The listing builds one solid part. Answer for the finished solid, in the listing's coordinates (mm). A direction names the side the tool comes from. Give positions to 0.01 mm unless a question says otherwise; leave off trailing zeros. Loops run counter-clockwise (first coordinate to the right, second up) from the corner with the lowest first, then second, coordinate; pieces in that order, holes last. Notation, with made-up numbers: (-14.75, 4) -> (22.25, 4) arc R13 ccw to (22.25, 25) -> close; hole circle Ø8 at (23, 9.5). An arc over 180 degrees is marked (long way). One line per question, with ' | ' between items. Start each with the question number.
from build123d import *
from OCP.BRepFilletAPI import BRepFilletAPI_MakeChamfer

# Parameters (mm, degrees)
SKETCH1_W           = 11.3
SKETCH1_H           = 9.85
BOSS_EXTRUDE1_DEPTH = 15.75
SKETCH2_W           = 0.45
SKETCH2_H           = 4
CUT_EXTRUDE1_DEPTH  = 15.75
SKETCH3_W           = 5.6
SKETCH3_H           = 3.18
CUT_EXTRUDE2_DEPTH  = 8.38
CHAMFER1_SIZE       = 0.38
CHAMFER1_SIZE2      = 0.219393102
CHAMFER2_SIZE       = 0.38
CHAMFER2_SIZE2      = 0.219393102
SKETCH4_W           = 1
SKETCH4_H           = 10.13
SKETCH4_H_2         = 8.63
BOSS_EXTRUDE2_DEPTH = 0.83
SKETCH5_W           = 1.2
SKETCH5_H           = 0.75
CUT_EXTRUDE3_DEPTH  = 19.829431749
SKETCH6_W           = 1.2
SKETCH6_H           = 6.44
CUT_EXTRUDE4_DEPTH  = 1.29
CUT_EXTRUDE5_DEPTH  = 2


with BuildPart() as part:
    # Sketch1 → Boss-Extrude1 (new body)
    with BuildSketch(Plane.XY.offset(-0.38)):
        with Locations((0, 5.325)):
            Rectangle(SKETCH1_W, SKETCH1_H)
    extrude(amount=-BOSS_EXTRUDE1_DEPTH)

    # Sketch2 → Cut-Extrude1 (cut)
    with BuildSketch(Plane(origin=(0, 10.25, 0), x_dir=(1, 0, 0), z_dir=(0, 1, 0))):
        with Locations((-5.425, 14.13)):
            Rectangle(SKETCH2_W, SKETCH2_H)
        with Locations((5.425, 14.13)):
            Rectangle(SKETCH2_W, SKETCH2_H)
    extrude(amount=-CUT_EXTRUDE1_DEPTH, mode=Mode.SUBTRACT)

    # Sketch3 → Cut-Extrude2 (cut)
    with BuildSketch(Plane.XY.offset(-0.38)):
        with BuildLine():
            Line((-4.225, 7.352598846), (-4.225, 6.45))
            Line((-4.225, 6.45), (-4.625, 6.45))
            Line((-4.625, 6.45), (-4.625, 2.45))
            Line((-4.625, 2.45), (-4.225, 2.45))
            Line((-4.225, 2.45), (-4.225, 1.74))
            ThreePointArc((-4.225, 1.74), (-4.113700577, 1.471299423), (-3.845, 1.36))
            Line((-3.845, 1.36), (3.845, 1.36))
            ThreePointArc((3.845, 1.36), (4.113700577, 1.471299423), (4.225, 1.74))
            Line((4.225, 1.74), (4.225, 2.45))
            Line((4.225, 2.45), (4.625, 2.45))
            Line((4.625, 2.45), (4.625, 6.45))
            Line((4.625, 6.45), (4.225, 6.45))
            Line((4.225, 6.45), (4.225, 7.352598846))
            ThreePointArc((4.225, 7.352598846), (4.196074222, 7.498018551), (4.113700577, 7.621299423))
            Line((4.113700577, 7.621299423), (2.706299423, 9.028700577))
            ThreePointArc((2.706299423, 9.028700577), (2.583018551, 9.111074222), (2.437598846, 9.14))
            Line((2.437598846, 9.14), (-2.437598846, 9.14))
            ThreePointArc((-2.437598846, 9.14), (-2.583018551, 9.111074222), (-2.706299423, 9.028700577))
            Line((-2.706299423, 9.028700577), (-4.113700577, 7.621299423))
            ThreePointArc((-4.113700577, 7.621299423), (-4.196074222, 7.498018551), (-4.225, 7.352598846))
        make_face()
        with Locations((0, 5.25)):
            Rectangle(SKETCH3_W, SKETCH3_H, mode=Mode.SUBTRACT)
    extrude(amount=-CUT_EXTRUDE2_DEPTH, mode=Mode.SUBTRACT)

    # Chamfer1: one chamfer whose edges measure the first distance from different faces: ONE call of the kernel's chamfer builder (chamfer() names one face for all edges)
    chamfer1_edges_1 = [part.edges().sort_by_distance(p)[0] for p in [
        (-2.8, 5.25, -0.38),
    ]]
    chamfer1_side_1 = [part.faces().sort_by_distance(p)[0] for p in [
        (-2.8, 5.25, -4.57),
    ]]
    chamfer1_edges_2 = [part.edges().sort_by_distance(p)[0] for p in [
        (0, 6.84, -0.38),
    ]]
    chamfer1_side_2 = [part.faces().sort_by_distance(p)[0] for p in [
        (0, 6.84, -4.57),
    ]]
    chamfer1_edges_3 = [part.edges().sort_by_distance(p)[0] for p in [
        (2.8, 5.25, -0.38),
    ]]
    chamfer1_side_3 = [part.faces().sort_by_distance(p)[0] for p in [
        (2.8, 5.25, -4.57),
    ]]
    chamfer1_edges_4 = [part.edges().sort_by_distance(p)[0] for p in [
        (0, 3.66, -0.38),
    ]]
    chamfer1_side_4 = [part.faces().sort_by_distance(p)[0] for p in [
        (0, 3.66, -4.57),
    ]]
    chamfer1 = BRepFilletAPI_MakeChamfer(part.part.solid().wrapped)
    for e in chamfer1_edges_1:
        chamfer1.Add(CHAMFER1_SIZE, CHAMFER1_SIZE2, e.wrapped, chamfer1_side_1[0].wrapped)  # the first distance lies on this face
    for e in chamfer1_edges_2:
        chamfer1.Add(CHAMFER1_SIZE, CHAMFER1_SIZE2, e.wrapped, chamfer1_side_2[0].wrapped)  # the first distance lies on this face
    for e in chamfer1_edges_3:
        chamfer1.Add(CHAMFER1_SIZE, CHAMFER1_SIZE2, e.wrapped, chamfer1_side_3[0].wrapped)  # the first distance lies on this face
    for e in chamfer1_edges_4:
        chamfer1.Add(CHAMFER1_SIZE, CHAMFER1_SIZE2, e.wrapped, chamfer1_side_4[0].wrapped)  # the first distance lies on this face
    add(Compound.cast(chamfer1.Shape()), mode=Mode.REPLACE)

    # Chamfer2: one chamfer whose edges measure the first distance from different faces: ONE call of the kernel's chamfer builder (chamfer() names one face for all edges)
    chamfer2_edges_1 = [part.edges().sort_by_distance(p)[0] for p in [
        (-4.196074222, 7.498018551, -0.38),
    ]]
    chamfer2_side_1 = [part.faces().sort_by_distance(p)[0] for p in [
        (-4.196074222, 7.498018551, -4.57),
    ]]
    chamfer2_edges_2 = [part.edges().sort_by_distance(p)[0] for p in [
        (-4.225, 6.901299423, -0.38),
    ]]
    chamfer2_side_2 = [part.faces().sort_by_distance(p)[0] for p in [
        (-4.225, 6.901299423, -4.57),
    ]]
    chamfer2_edges_3 = [part.edges().sort_by_distance(p)[0] for p in [
        (-4.225, 2.095, -0.38),
    ]]
    chamfer2_side_3 = [part.faces().sort_by_distance(p)[0] for p in [
        (-4.225, 2.095, -4.57),
    ]]
    chamfer2_edges_4 = [part.edges().sort_by_distance(p)[0] for p in [
        (-4.113700577, 1.471299423, -0.38),
    ]]
    chamfer2_side_4 = [part.faces().sort_by_distance(p)[0] for p in [
        (-4.113700577, 1.471299423, -4.57),
    ]]
    chamfer2_edges_5 = [part.edges().sort_by_distance(p)[0] for p in [
        (0, 1.36, -0.38),
    ]]
    chamfer2_side_5 = [part.faces().sort_by_distance(p)[0] for p in [
        (0, 1.36, -4.57),
    ]]
    chamfer2_edges_6 = [part.edges().sort_by_distance(p)[0] for p in [
        (4.113700577, 1.471299423, -0.38),
    ]]
    chamfer2_side_6 = [part.faces().sort_by_distance(p)[0] for p in [
        (4.113700577, 1.471299423, -4.57),
    ]]
    chamfer2_edges_7 = [part.edges().sort_by_distance(p)[0] for p in [
        (4.225, 2.095, -0.38),
    ]]
    chamfer2_side_7 = [part.faces().sort_by_distance(p)[0] for p in [
        (4.225, 2.095, -4.57),
    ]]
    chamfer2_edges_8 = [part.edges().sort_by_distance(p)[0] for p in [
        (4.225, 6.901299423, -0.38),
    ]]
    chamfer2_side_8 = [part.faces().sort_by_distance(p)[0] for p in [
        (4.225, 6.901299423, -4.57),
    ]]
    chamfer2_edges_9 = [part.edges().sort_by_distance(p)[0] for p in [
        (4.196074222, 7.498018551, -0.38),
    ]]
    chamfer2_side_9 = [part.faces().sort_by_distance(p)[0] for p in [
        (4.196074222, 7.498018551, -4.57),
    ]]
    chamfer2_edges_10 = [part.edges().sort_by_distance(p)[0] for p in [
        (3.41, 8.325, -0.38),
    ]]
    chamfer2_side_10 = [part.faces().sort_by_distance(p)[0] for p in [
        (3.41, 8.325, -4.57),
    ]]
    chamfer2_edges_11 = [part.edges().sort_by_distance(p)[0] for p in [
        (2.583018551, 9.111074222, -0.38),
    ]]
    chamfer2_side_11 = [part.faces().sort_by_distance(p)[0] for p in [
        (2.583018551, 9.111074222, -4.57),
    ]]
    chamfer2_edges_12 = [part.edges().sort_by_distance(p)[0] for p in [
        (0, 9.14, -0.38),
    ]]
    chamfer2_side_12 = [part.faces().sort_by_distance(p)[0] for p in [
        (0, 9.14, -4.57),
    ]]
    chamfer2_edges_13 = [part.edges().sort_by_distance(p)[0] for p in [
        (-2.583018551, 9.111074222, -0.38),
    ]]
    chamfer2_side_13 = [part.faces().sort_by_distance(p)[0] for p in [
        (-2.583018551, 9.111074222, -4.57),
    ]]
    chamfer2_edges_14 = [part.edges().sort_by_distance(p)[0] for p in [
        (-3.41, 8.325, -0.38),
    ]]
    chamfer2_side_14 = [part.faces().sort_by_distance(p)[0] for p in [
        (-3.41, 8.325, -4.57),
    ]]
    chamfer2 = BRepFilletAPI_MakeChamfer(part.part.solid().wrapped)
    for e in chamfer2_edges_1:
        chamfer2.Add(CHAMFER2_SIZE, CHAMFER2_SIZE2, e.wrapped, chamfer2_side_1[0].wrapped)  # the first distance lies on this face
    for e in chamfer2_edges_2:
        chamfer2.Add(CHAMFER2_SIZE, CHAMFER2_SIZE2, e.wrapped, chamfer2_side_2[0].wrapped)  # the first distance lies on this face
    for e in chamfer2_edges_3:
        chamfer2.Add(CHAMFER2_SIZE, CHAMFER2_SIZE2, e.wrapped, chamfer2_side_3[0].wrapped)  # the first distance lies on this face
    for e in chamfer2_edges_4:
        chamfer2.Add(CHAMFER2_SIZE, CHAMFER2_SIZE2, e.wrapped, chamfer2_side_4[0].wrapped)  # the first distance lies on this face
    for e in chamfer2_edges_5:
        chamfer2.Add(CHAMFER2_SIZE, CHAMFER2_SIZE2, e.wrapped, chamfer2_side_5[0].wrapped)  # the first distance lies on this face
    for e in chamfer2_edges_6:
        chamfer2.Add(CHAMFER2_SIZE, CHAMFER2_SIZE2, e.wrapped, chamfer2_side_6[0].wrapped)  # the first distance lies on this face
    for e in chamfer2_edges_7:
        chamfer2.Add(CHAMFER2_SIZE, CHAMFER2_SIZE2, e.wrapped, chamfer2_side_7[0].wrapped)  # the first distance lies on this face
    for e in chamfer2_edges_8:
        chamfer2.Add(CHAMFER2_SIZE, CHAMFER2_SIZE2, e.wrapped, chamfer2_side_8[0].wrapped)  # the first distance lies on this face
    for e in chamfer2_edges_9:
        chamfer2.Add(CHAMFER2_SIZE, CHAMFER2_SIZE2, e.wrapped, chamfer2_side_9[0].wrapped)  # the first distance lies on this face
    for e in chamfer2_edges_10:
        chamfer2.Add(CHAMFER2_SIZE, CHAMFER2_SIZE2, e.wrapped, chamfer2_side_10[0].wrapped)  # the first distance lies on this face
    for e in chamfer2_edges_11:
        chamfer2.Add(CHAMFER2_SIZE, CHAMFER2_SIZE2, e.wrapped, chamfer2_side_11[0].wrapped)  # the first distance lies on this face
    for e in chamfer2_edges_12:
        chamfer2.Add(CHAMFER2_SIZE, CHAMFER2_SIZE2, e.wrapped, chamfer2_side_12[0].wrapped)  # the first distance lies on this face
    for e in chamfer2_edges_13:
        chamfer2.Add(CHAMFER2_SIZE, CHAMFER2_SIZE2, e.wrapped, chamfer2_side_13[0].wrapped)  # the first distance lies on this face
    for e in chamfer2_edges_14:
        chamfer2.Add(CHAMFER2_SIZE, CHAMFER2_SIZE2, e.wrapped, chamfer2_side_14[0].wrapped)  # the first distance lies on this face
    add(Compound.cast(chamfer2.Shape()), mode=Mode.REPLACE)

    # Sketch4 → Boss-Extrude2 (add)
    with BuildSketch(Plane(origin=(0, 0.4, 0), x_dir=(-1, 0, 0), z_dir=(0, -1, 0))):
        with Locations((3.75, 11.065)):
            Rectangle(SKETCH4_W, SKETCH4_H)
        with Locations((0, 11.815)):
            Rectangle(SKETCH4_W, SKETCH4_H_2)
        with Locations((-3.75, 11.065)):
            Rectangle(SKETCH4_W, SKETCH4_H)
    extrude(amount=BOSS_EXTRUDE2_DEPTH)

    # Sketch5 → Cut-Extrude3 (cut, through all)
    with BuildSketch(Plane.XY.offset(-1.38)):
        with Locations((-1.25, 6.465)):
            Rectangle(SKETCH5_W, SKETCH5_H)
        with Locations((1.25, 6.465)):
            Rectangle(SKETCH5_W, SKETCH5_H)
        with Locations((1.25, 4.035)):
            Rectangle(SKETCH5_W, SKETCH5_H)
        with Locations((-1.25, 4.035)):
            Rectangle(SKETCH5_W, SKETCH5_H)
    extrude(amount=-CUT_EXTRUDE3_DEPTH, mode=Mode.SUBTRACT)

    # Sketch6 → Cut-Extrude4 (cut)
    with BuildSketch(Plane(origin=(0, 0, -16.13), x_dir=(-1, 0, 0), z_dir=(0, 0, -1))):
        with Locations((-1.25, 3.62)):
            Rectangle(SKETCH6_W, SKETCH6_H)
        with Locations((1.25, 3.62)):
            Rectangle(SKETCH6_W, SKETCH6_H)
    extrude(amount=-CUT_EXTRUDE4_DEPTH, mode=Mode.SUBTRACT)

    # Sketch7 → Cut-Extrude5 (cut)
    with BuildSketch(Plane(origin=(0, 0, -14.84), x_dir=(-1, 0, 0), z_dir=(0, 0, -1))):
        Polygon((-1.55, 2.66), (-1.55, 0), (-0.95, 0), (-0.95, 2.66), (-0.65, 2.66), (-0.65, 4.41), (-1.85, 4.41), (-1.85, 2.66), align=None)
        Polygon((0.95, 2.66), (0.95, 0), (1.55, 0), (1.55, 2.66), (1.85, 2.66), (1.85, 4.41), (0.65, 4.41), (0.65, 2.66), align=None)
    extrude(amount=-CUT_EXTRUDE5_DEPTH, mode=Mode.SUBTRACT)


solid = part.part
1. The part is cut by section B-B (z = -12.5). Count the separate pieces of the cut face and the enclosed holes in it, plus the area to 3 significant figures.
2. The part is cut by section A-A (y = 5.25). Write down the section's boundary in (x, z) (3 decimals).
3. Determine the mould class of faces 5 (the flat face through (4, -0.43, -11)), 6 (the flat face through (4, 0, -6)), 7 (the flat face through (-1.2, 2.4, -12.84)) for opening direction Y: released by +Y, released by -Y, zero draft, split by the parting line, or undercut.
4. Each of these flat-tipped pins is pushed along its axis until it touches: pin 1 Ø3 at (y, z) = (1, -14.5) entering from -X; pin 2 Ø1 at (x, z) = (-1.5, -10.5) entering from -Y; pin 3 Ø0.7 at (y, z) = (0, -12) entering from -X. Where does it stop, or does it pass through?
5. For faces 1 (the flat face through (0, 0, -7.5)), 2 (the flat face through (-1, 6.09, -8)), 3 (the flat face through (-1.55, 2, -14)), 4 (the flat face through (-0.5, 0, -12)), determine the directions among +Z, -Z, +X, -X, +Y, -Y from which every point of the face is accessible in a straight line to the end or side of a thin tool.
6. Straight lines are drawn through the part: L1, parallel to X at y = 1.5, z = -14.5; L2, parallel to X at y = 6.5, z = -9.75; L3, parallel to Y at x = -2, z = -1.5. For each, find the intervals that lie inside material, in ascending order.
Check sheet entries:
1) separate pieces: 1 | enclosed holes: 4 | area: 101 mm^2
2) outline: (-5.65, -12.13) -> (-5.2, -12.13) -> (-5.2, -16.13) -> (-1.85, -16.13) -> (-1.85, -14.84) -> (-0.65, -14.84) -> (-0.65, -16.13) -> (0.65, -16.13) -> (0.65, -14.84) -> (1.85, -14.84) -> (1.85, -16.13) -> (5.2, -16.13) -> (5.2, -12.13) -> (5.65, -12.13) -> (5.65, -0.38) -> (4.625, -0.38) -> (4.625, -8.76) -> (2.8, -8.76) -> (2.8, -0.76) -> (2.581, -0.38) -> (-2.581, -0.38) -> (-2.8, -0.76) -> (-2.8, -8.76) -> (-4.625, -8.76) -> (-4.625, -0.38) -> (-5.65, -0.38) -> close
3) face 5: released by -Y | face 6: zero draft | face 7: undercut
4) pin 1: stops at x = -5.2 | pin 2: stops at y = 0.4 | pin 3: stops at x = -4.25
5) face 1: +Z, -Y | face 2: -Z | face 3: -Z, -Y | face 4: +Z, -Z, -Y
6) L1: x = -5.2 to -1.55, -0.95 to 0.95, 1.55 to 5.2 | L2: x = -5.65 to -1.85, -0.65 to 0.65, 1.85 to 5.65 | L3: y = 0.4 to 1.36, 3.66 to 6.84, 9.14 to 10.25
